Geometry check sheet. Reference: the model listing, model coordinates, mm. Face numbers are marked on the shaded views. A direction names the side the tool comes from. Round coordinates to 2 decimals unless told otherwise and drop trailing zeros. Write each loop counter-clockwise with the first axis right and the second up, starting at its lowest first coordinate (ties: lowest second). Pieces come first, ordered by that corner, then holes.
from build123d import *

# Parameters (mm, degrees)
F0_W           = 51.2767769396
F0_H           = 40.3746776283
F1_DEPTH       = 25.4
F2_W           = 14.1758769751
F2_H           = 15.7698839903
F3_DEPTH       = 12.7
F4_T           = -2.54
F5_SIZE        = 2.53999
F7_D           = 2.54
F7_CBORE_D     = 5.08
F7_CBORE_DEPTH = 2.54


# Not quite as in the source:
# - a fillet or chamfer is up to 0.001 mm smaller than in the source, because OpenCascade refuses the exact size


with BuildPart() as f1:
    # F0 (on Top) → F1 (new body)
    with BuildSketch(Plane.XY):
        with Locations((25.6383884698, 20.1873388141)):
            Rectangle(F0_W, F0_H)
    extrude(amount=F1_DEPTH)

    # F2 (on face) → F3 (join)
    with BuildSketch(Plane.XY.offset(25.4)):
        with Locations((19.3085148931, 20.5943360925)):
            Rectangle(F2_W, F2_H)
    extrude(amount=-F3_DEPTH)

    # F4
    f4_openings = [f1.faces().sort_by_distance(p)[0] for p in [
        (25.638388, 20.187339, 0),
    ]]
    offset(amount=F4_T, openings=f4_openings)

    # F5 (size 2.54 in the source; OpenCascade refuses exactly that, so slightly less here)
    f5_edges = [f1.edges().sort_by_distance(p)[0] for p in [
        (2.54, 20.187339, 0),
        (25.638388, 37.834678, 0),
        (48.736777, 20.187339, 0),
        (25.638388, 2.54, 0),
    ]]
    chamfer(f5_edges, length=F5_SIZE)

    # F7 (through all)
    with Locations(Plane(origin=(0, 0, 22.86), x_dir=(1, 0, 0), z_dir=(0, 0, -1))):
        with Locations((28.0292164534, -20.6155125052)):
            CounterBoreHole(F7_D / 2, F7_CBORE_D / 2, F7_CBORE_DEPTH)


solid = f1.part
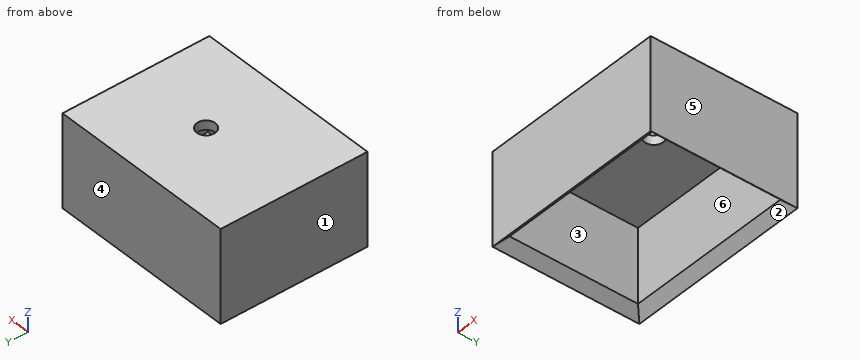
1. Scan lines: line 1 along Y through (x, z) = (5, 14); line 2 along X through (y, z) = (6, 9); line 3 along Z through (x, y) = (19, 15). Record each from-to range of solid material in increasing order.
2. Section check A-A (z = 19.5). Record the cut outline in (x, y), plus the area to 3 significant figures.
3. Depth check by flat-ended pin: pin 1 Ø1.5 at (x, y) = (13, 29.5) entering from -Z; pin 2 Ø3 at (x, y) = (28.03, 20.62) entering from -Z. Enter the tip coordinate at first touch or a pass-through.
4. Access from +Z, -Z, +X, -X, +Y, -Y to the whole of each face (thin tool, end or side, straight path). Record for the marked faces 1 and 2.
5. Release check for a two-part mould opening along X. For the marked faces 3, 4, 5 and 6 record: +X half, -X half, draft (parallel to the pull), parting line (faces both ways), or undercut.
Results below:
1. line 1: y = 0 to 2.54, 37.83 to 40.37
1. line 2: x = 0 to 2.54, 48.74 to 51.28
1. line 3: z = 22.86 to 25.4
2. outline: (0, 0) - (51.28, 0) - (51.28, 40.37) - (0, 40.37) - close; hole (2.54, 2.54) - (48.74, 2.54) - (48.74, 37.83) - (2.54, 37.83) - close
2. area: 440 mm2
3. pin 1: stops at z = 22.86
3. pin 2: passes through
4. face 1: +Z, -Z, -X, +Y, -Y
4. face 2: -Z
5. face 3: undercut
5. face 4: draft
5. face 5: +X half
5. face 6: undercut
